Model file for the job. Use its own axes, mm. A direction names the side the tool comes from. Give positions to 0.01 mm unless a question says otherwise; leave off trailing zeros. Order: outer loops, then holes, each group sorted by start corner. A loop starts at its lowest first (then second) coordinate and runs counter-clockwise, first axis right, second up. Notation, with made-up numbers: M -28,80.25 L -8,80.25 A19 ccw -8,112.25 Z; hole C -24.5,-5.75 d4. An arc over 180 degrees is marked long. Return JSON: item names as keys, results as strings. Group by question number.
1. Slice it at B-B on x = -39. List the corners of the cut face in (y, z), then the cut area to 3 significant figures.
2. Slice it at C-C on y = 0. List the corners of the cut face in (x, z).
3. 3-axis set-ups, long thin cutter, end or side, ignore diameter. For faces 1 (the face through (45.25, 19, 30)), 2 (the face through (-41, 19, 2)): which of +Z, -Z, +X, -X, +Y, -Y reach the whole face in a straight line?
4. Slice it at A-A on z = 14.5. List the corners of the cut face in (x, y), then the cut area to 3 significant figures.
5. Slice it at D-D on x = 37.25. List the corners of the cut face in (y, z), then the cut area to 3 significant figures.
6. Pin check, flat tips, straight feed: pin 1 (2 mm diameter, centred on x = 7, y = 14.5, fed in from +Z); pin 2 (2.5 mm diameter, centred on x = -39, y = -24.5, fed in from +Z); pin 3 (8 mm diameter, centred on x = -15, y = -11, fed in from -Z). Stop position of each tip, or through.
7. Wall check: probe 1 along X at (y, z) = (-13, 35.5); probe 2 along X at (y, z) = (-24, 1); probe 3 along X at (y, z) = (-23, 1). Give the ranges that are in metal, low to high. Write a range as [from, to].
8. Two-plate mould, pull along X, no slides. Class faces 3 (the face through (43.25, 19, 30)), 4 (the face through (-39, 68, 1)), 5 (the face through (-124.75, 19, 30)): released by +X, released by -X, zero draft, split by the parting line, or undercut.
from build123d import *

# Parameters (mm, degrees)
PAD002_DEPTH    = 250
PAD003_DEPTH    = 150
SKETCH_W        = 170
SKETCH_H        = 100
PAD_DEPTH       = 60
FILLET_R        = 3
SKETCH001_W     = 17
SKETCH001_H     = 14.3
SKETCH001_W_2   = 15.6
SKETCH001_H_2   = 16.5
POCKET_DEPTH    = 45.251
SKETCH002_W     = 8.2
SKETCH002_H     = 4.6
POCKET001_DEPTH = 30.001
SKETCH006_W     = 165
SKETCH006_H     = 92
POCKET003_DEPTH = 500
SKETCH007_R     = 2.2
SKETCH007_R_2   = 1.75
POCKET004_DEPTH = 5


with BuildPart() as bottom_mask:
    # Sketch004 → Pad002 (new body, symmetric)
    with BuildSketch(Plane.XZ):
        with BuildLine():
            Line((-122.75, 60), (-122.75, 2.999996))
            ThreePointArc((-122.75, 2.999996), (-122.457105, 2.292892), (-121.75, 2))
            Line((-121.75, 2), (42.25, 2))
            ThreePointArc((42.25, 2), (42.957105, 2.292892), (43.25, 2.999996))
            Line((43.25, 2.999996), (43.25, 60))
            Line((43.25, 60), (-122.75, 60))
        make_face()
    extrude(amount=PAD002_DEPTH, both=True)

    # Sketch008 → Pad003 (join, symmetric)
    with BuildSketch(Plane.YZ):
        Polygon((-30, 60), (-30, 0), (-28, 0), (-28, 58), (68, 58), (68, 0), (70, 0), (70, 60), align=None)
    extrude(amount=PAD003_DEPTH, both=True)


with BuildPart() as bottom:
    # Sketch → Pad (new body)
    with BuildSketch(Plane.XY):
        with Locations((-39.75, 20)):
            Rectangle(SKETCH_W, SKETCH_H)
    extrude(amount=PAD_DEPTH)

    # Fillet
    fillet_edges = [bottom.edges().sort_by_distance(p)[0] for p in [
        (45.25, 20, 0),
        (-39.75, -30, 60),
        (-39.75, 70, 60),
        (-124.75, 20, 0),
    ]]
    fillet(fillet_edges, radius=FILLET_R)

    # Sketch001 → Pocket (cut, through all)
    with BuildSketch(Plane.YZ):
        with Locations((-17.8, 14.75)):
            Rectangle(SKETCH001_W, SKETCH001_H)
        with Locations((1.05, 16.2)):
            Rectangle(SKETCH001_W_2, SKETCH001_H_2)
        with Locations((19, 16.2)):
            Rectangle(SKETCH001_W_2, SKETCH001_H_2)
    extrude(amount=POCKET_DEPTH, mode=Mode.SUBTRACT)

    # Sketch002 → Pocket001 (cut, through all)
    with BuildSketch(Plane.XZ):
        with BuildLine():
            ThreePointArc((-34.67, 11.2), (-35.73066, 10.76066), (-36.17, 9.7))
            Line((-36.17, 8.74), (-36.17, 9.7))
            ThreePointArc((-36.17, 8.74), (-35.73066, 7.67934), (-34.67, 7.24))
            Line((-27.93, 7.24), (-34.67, 7.24))
            ThreePointArc((-27.93, 7.24), (-26.86934, 7.67934), (-26.43, 8.74))
            Line((-26.43, 9.7), (-26.43, 8.74))
            ThreePointArc((-26.43, 9.7), (-26.86934, 10.76066), (-27.93, 11.2))
            Line((-34.67, 11.2), (-27.93, 11.2))
        make_face()
        with Locations((-16.704733, 9.1)):
            Rectangle(SKETCH002_W, SKETCH002_H)
        with Locations((-3.304733, 9.1)):
            Rectangle(SKETCH002_W, SKETCH002_H)
    extrude(amount=POCKET001_DEPTH, mode=Mode.SUBTRACT)

    # Sketch006 → Pocket003 (cut)
    with BuildSketch(Plane.XY.offset(30)):
        with Locations((-39.75, 20)):
            Rectangle(SKETCH006_W, SKETCH006_H)
    extrude(amount=POCKET003_DEPTH, mode=Mode.SUBTRACT)

    # Sketch007 → Pocket004 (cut)
    with BuildSketch(Plane.XY):
        with Locations((-39, 24.5)):
            Circle(SKETCH007_R)
        with Locations((19, 24.5)):
            Circle(SKETCH007_R)
        with Locations((-39, -24.5)):
            Circle(SKETCH007_R)
        with Locations((19, -24.5)):
            Circle(SKETCH007_R)
        with Locations((-112, 18.5)):
            Circle(SKETCH007_R)
        with Locations((-116.75, -23.9)):
            Circle(SKETCH007_R_2)
        with Locations((-116.75, 63.9)):
            Circle(SKETCH007_R_2)
        with Locations((37.25, 63.9)):
            Circle(SKETCH007_R_2)
    extrude(amount=POCKET004_DEPTH, mode=Mode.SUBTRACT)

    # Cut001: cut Bottom Mask
    add(bottom_mask.part, mode=Mode.SUBTRACT)


solid = bottom.part
Result:
{
 "1": {"outline": "M -28,0 L -26.7,0 L -26.7,2 L -28,2 Z; M -22.3,0 L 22.3,0 L 22.3,2 L -22.3,2 Z; M 26.7,0 L 68,0 L 68,2 L 26.7,2 Z", "area": "174 mm2"},
 "2": {"outline": "M -124.75,3 A3 ccw -121.75,0 L 42.25,0 A3 ccw 45.25,3 L 45.25,7.95 L 43.25,7.95 L 43.25,3 A1 cw 42.25,2 L -121.75,2 A1 cw -122.75,3 L -122.75,58 L -124.75,58 Z; M 43.25,24.45 L 45.25,24.45 L 45.25,58 L 43.25,58 Z"},
 "3": {"face 1": "+Z, -Z, +X, +Y, -Y", "face 2": "+Z, +Y, -Y"},
 "4": {"outline": "M -124.75,-28 L -122.75,-28 L -122.75,68 L -124.75,68 Z; M 43.25,-28 L 45.25,-28 L 45.25,-26.3 L 43.25,-26.3 Z; M 43.25,-9.3 L 45.25,-9.3 L 45.25,-6.75 L 43.25,-6.75 Z; M 43.25,8.85 L 45.25,8.85 L 45.25,11.2 L 43.25,11.2 Z; M 43.25,26.8 L 45.25,26.8 L 45.25,68 L 43.25,68 Z", "area": "288 mm2"},
 "5": {"outline": "M -28,0 L 62.15,0 L 62.15,2 L -28,2 Z; M 65.65,0 L 68,0 L 68,2 L 65.65,2 Z", "area": "185 mm2"},
 "6": {"pin 1": "stops at z = 2", "pin 2": "passes through", "pin 3": "stops at z = 0"},
 "7": {"probe 1": "x = [-124.75, -122.75], [43.25, 45.25]", "probe 2": "x = [-123.99, -118.5], [-115, -41.14], [-36.86, 16.86], [21.14, 44.49]", "probe 3": "x = [-123.99, -118.25], [-115.25, -40.61], [-37.39, 17.39], [20.61, 44.49]"},
 "8": {"face 3": "undercut", "face 4": "zero draft", "face 5": "released by -X"}
}
